```python
from build123d import *

# Parameters (mm, degrees)
F0_R     = 26
F1_DEPTH = 105
F2_R     = 10
F3_DEPTH = 37
F7_START = -5
F7_DEPTH = 50
F8_R     = 3
F9_DEPTH = 45.0490971485


with BuildPart() as f1:
    # F0 (on Top) → F1 (new body)
    with BuildSketch(Plane.XY):
        Circle(F0_R)
    extrude(amount=F1_DEPTH)

    # F2 (on face) → F3 (join)
    with BuildSketch(Plane(origin=(0, 0, 0), x_dir=(1, 0, 0), z_dir=(0, 0, -1))):
        Circle(F2_R)
    extrude(amount=F3_DEPTH)

    # F4 (on Right) → F5 (revolve)
    with BuildSketch(Plane.YZ):
        Polygon((0, -52), (0, -37), (-1.58, -37), (-1.58, -43.039374725), align=None)
    revolve(axis=Axis((0, 0, -44.5), (0, 0, -1)))

    # F6 (on face) → F7 (join)
    with BuildSketch(Plane(origin=(0, 0, 0), x_dir=(1, 0, 0), z_dir=(0, 0, -1)).offset(F7_START)):
        with BuildLine():
            Line((-45, -8.9544598013), (-31.2420813914, -8.9544598013))
            ThreePointArc((-31.2420813914, -8.9544598013), (0, -32.5), (31.2420813914, -8.9544598013))
            Line((31.2420813914, -8.9544598013), (45, -8.9544598013))
            Line((45, -8.9544598013), (45, 36.0936373472))
            Line((45, 36.0936373472), (-45, 36.0936373472))
            Line((-45, 36.0936373472), (-45, -8.9544598013))
        make_face()
    extrude(amount=-F7_DEPTH)

    # F8 (on face) → F9 (cut, through all)
    with BuildSketch(Plane(origin=(0, 8.9544598013, 0), x_dir=(-1, 0, 0), z_dir=(0, 1, 0))):
        with Locations((-39, 49)):
            Circle(F8_R)
        with Locations((-39, 11)):
            Circle(F8_R)
        with Locations((39, 49)):
            Circle(F8_R)
        with Locations((39, 11)):
            Circle(F8_R)
    extrude(amount=-F9_DEPTH, mode=Mode.SUBTRACT)


solid = f1.part
```
Could you check a few things on this model? Use its own coordinates, in mm. A direction names the side the tool comes from. Round coordinates to 2 decimals unless told otherwise and drop trailing zeros. Loops run counter-clockwise (first coordinate to the right, second up) from the corner with the lowest first, then second, coordinate; pieces in that order, holes last. Notation, with made-up numbers: (39, 68) - (45, 68) arc R13 ccw to (45, 83) - close; hole circle Ø1 at (30.5, 77). An arc over 180 degrees is marked (long way). Answer in a Markdown table with one row per item. Add a question column.
(1) If we section it at A-A (z = 49): Please give me the cut outline in (x, y).
(2) For faces 1 (the face through (-38, 8.954, 30)), 2 (the face through (9, -25, 55)), 3 (the face through (0, 0, 105)), 4 (the face through (11, 0, 0)), which set-ups out of +Z, -Z, +X, -X, +Y, -Y let a thin tool reach every point of the face, with its end or its side?
(3) I need wall thicknesses on line 1 along Z through (x, y) = (-39, -14); line 2 along X through (y, z) = (7.5, 47); line 3 along Z through (x, y) = (18.5, -28). Which ranges of each line are inside material? Lowest first, please.
(4) If we section it at C-C (y = -13): Please give me the cut outline in (x, z).
(5) I'm going to push flat-ended pins straight in: pin 1 (4 mm diameter, centred on x = -2.5, z = 68, fed in from -Y); pin 2 (8 mm diameter, centred on x = 39, z = 49, fed in from +Y); pin 3 (5 mm diameter, centred on x = -35.5, y = -14, fed in from +Z). Where does each tip first touch, or does it pass through?
(6) If we mould it in two halves opening along X, with no side actions, what happens to faces 5 (the face through (38, 8.954, 30)), 6 (the face through (-36, -13, 11)), 7 (the face through (-20.633, -15.821, 79.65))? For each: pulls with the +X half, pulls with the -X half, needs draft (parallel to the pull), parting line crosses it, or undercut.
(7) If we section it at B-B (x = 39): Please give me the cut outline in (y, z).
(8) If we section it at D-D (y = 19.5): Please give me the cut outline in (x, z), plus the area to 3 significant figures.
Model answer:
| question | item | result |
|---|---|---|
| 1 | outline | (-45, -36.09) - (-42, -36.09) - (-42, 8.95) - (-45, 8.95) - close; (-36, -36.09) - (36, -36.09) - (36, 8.95) - (31.24, 8.95) arc R32.5 ccw to (-31.24, 8.95) - (-36, 8.95) - close; (42, -36.09) - (45, -36.09) - (45, 8.95) - (42, 8.95) - close |
| 2 | face 1 | +Z, -Z, -X, +Y |
| 2 | face 2 | +Z |
| 2 | face 3 | +Z, +X, -X, +Y, -Y |
| 2 | face 4 | -Z |
| 3 | line 1 | z = 5 to 8, 14 to 46, 52 to 55 |
| 3 | line 2 | x = -45 to -41.24, -36.76 to 36.76, 41.24 to 45 |
| 3 | line 3 | z = 5 to 55 |
| 4 | outline | (-45, 5) - (-22.52, 5) - (-22.52, 0) - (22.52, 0) - (22.52, 5) - (45, 5) - (45, 55) - (22.52, 55) - (22.52, 105) - (-22.52, 105) - (-22.52, 55) - (-45, 55) - close; hole circle Ø6 at (-39, 11); hole circle Ø6 at (-39, 49); hole circle Ø6 at (39, 11); hole circle Ø6 at (39, 49) |
| 5 | pin 1 | stops at y = -26 |
| 5 | pin 2 | stops at y = 8.95 |
| 5 | pin 3 | stops at z = 55 |
| 6 | face 5 | needs draft |
| 6 | face 6 | undercut |
| 6 | face 7 | parting line crosses it |
| 7 | outline | (-36.09, 5) - (8.95, 5) - (8.95, 8) - (-36.09, 8) - close; (-36.09, 14) - (8.95, 14) - (8.95, 46) - (-36.09, 46) - close; (-36.09, 52) - (8.95, 52) - (8.95, 55) - (-36.09, 55) - close |
| 8 | outline | (-26, 5) - (-17.2, 5) - (-17.2, 0) - (17.2, 0) - (17.2, 5) - (26, 5) - (26, 55) - (17.2, 55) - (17.2, 105) - (-17.2, 105) - (-17.2, 55) - (-26, 55) - close |
| 8 | area | 4,490 mm² |
